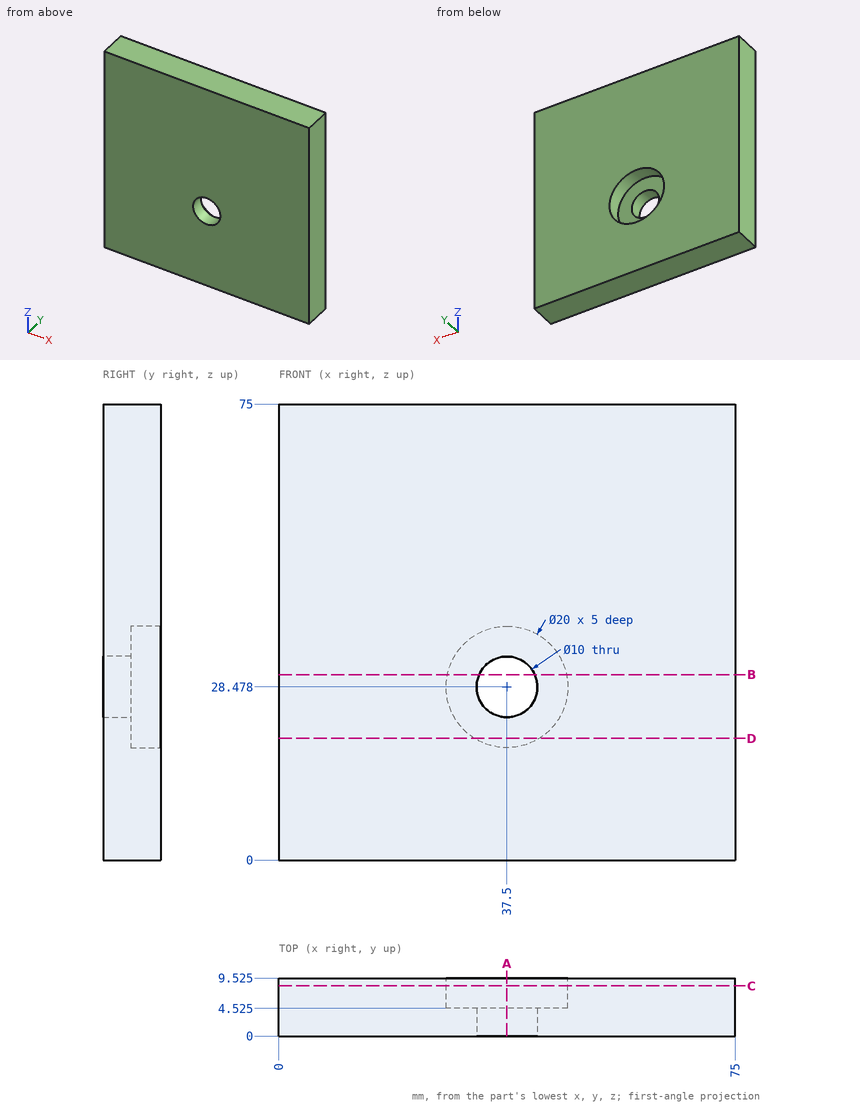
Can you work these out from the drawing? Everything is in mm from the part's minimum corner. Coordinates: 2 decimals unless noted, no trailing zeros. Loops run counter-clockwise (first coordinate to the right, second up) from the corner with the lowest first, then second, coordinate; pieces in that order, holes last. Notation, with made-up numbers: (-15, 41.25) - (-4, 41.25) arc R33 ccw to (-4, 79.25) - close; hole circle Ø6 at (70.5, 58.25). An arc over 180 degrees is marked (long way). Use a Markdown table: item, result.
Item 1: I want a section at D-D on z = 20. Please give me the cut outline in (x, y) (1 decimal).
Numbers:
| item | result |
|---|---|
| outline | (0, 0) - (75, 0) - (75, 9.5) - (42.8, 9.5) - (42.8, 4.5) - (32.2, 4.5) - (32.2, 9.5) - (0, 9.5) - close |
Item 2: If I drill on probe 1 along Z at (x, y) = (37.5, 1.3); probe 2 along X at (y, z) = (3, 26.5); probe 3 along X at (y, z) = (6, 26), over which ranges is the centre line in solid material (lowest first)? Write a range as from..to.
Numbers:
| item | result |
|---|---|
| probe 1 | z = 0..23.48, 33.48..75 |
| probe 2 | x = 0..32.91, 42.09..75 |
| probe 3 | x = 0..27.81, 47.19..75 |
Item 3: Will these pins go through, and if not, where does the flat tip stop? pin 1 (6 mm diameter, centred on x = 37.5, z = 28.48, fed in from -Y); pin 2 (10 mm diameter, centred on x = 63.5, z = 23, fed in from -Y).
Numbers:
| item | result |
|---|---|
| pin 1 | passes through |
| pin 2 | stops at y = 0 |
Item 4: I want a section at C-C on y = 8.25. Please give me the cut outline in (x, z), and give its area (3 significant figures).
Numbers:
| item | result |
|---|---|
| outline | (0, 0) - (75, 0) - (75, 75) - (0, 75) - close; hole circle Ø20 at (37.5, 28.48) |
| area | 5,310 mm2 |
Item 5: I want a section at B-B on z = 30.5. Please give me the cut outline in (x, y) (1 decimal), and give its area (3 significant figures).
Numbers:
| item | result |
|---|---|
| outline | (0, 0) - (32.9, 0) - (32.9, 4.5) - (27.7, 4.5) - (27.7, 9.5) - (0, 9.5) - close; (42.1, 0) - (75, 0) - (75, 9.5) - (47.3, 9.5) - (47.3, 4.5) - (42.1, 4.5) - close |
| area | 575 mm2 |
Item 6: I want a section at A-A on x = 37.5. Please give me the cut outline in (y, z) (1 decimal), and give its area (3 significant figures).
Numbers:
| item | result |
|---|---|
| outline | (0, 0) - (9.5, 0) - (9.5, 18.5) - (4.5, 18.5) - (4.5, 23.5) - (0, 23.5) - close; (0, 33.5) - (4.5, 33.5) - (4.5, 38.5) - (9.5, 38.5) - (9.5, 75) - (0, 75) - close |
| area | 569 mm2 |
